Build history of the part. All positions in model axes, mm. Face numbers are marked on the shaded views. A direction names the side the tool comes from. Round coordinates to 2 decimals unless told otherwise and drop trailing zeros. Write each loop counter-clockwise with the first axis right and the second up, starting at its lowest first coordinate (ties: lowest second). Pieces come first, ordered by that corner, then holes. Notation, with made-up numbers: (20.25, -7) - (44.25, -7) arc R33 ccw to (44.25, 30) - close; hole circle Ø2 at (29, -29). An arc over 180 degrees is marked (long way). Answer as a JSON object with one key per item and string values. Group by question number.
Item 1: Flat gauge pins, fed straight in: pin 1 (6 mm diameter, centred on x = -10, y = -7, fed in from +Z); pin 2 (5 mm diameter, centred on x = 11, y = 5, fed in from +Z); pin 3 (12 mm diameter, centred on x = -1, y = -9.5, fed in from +Z). Where does each tip first touch, or does it go through?
Item 2: Two-plate mould, pull along X, no slides. Class the marked faces 1, 2, 3 and 4: +X half, -X half, draft (parallel to the pull), parting line (faces both ways), or undercut.
Item 3: Probe line 1 (X direction, y = 7, z = 1.7); line 2 (Y direction, x = 10, z = 0.95); line 3 (Z direction, x = 0, y = -7.5). List the from-to ranges inside material, lowest first. Write a range as from..to.
Item 4: Slice it at C-C, the plane x = 10. List the corners of the cut face in (y, z), then the cut area to 3 significant figures.
Item 5: Slice it at B-B, the plane x = 0. List the corners of the cut face in (y, z), then the cut area to 3 significant figures.
Item 6: Which spindle directions (+Z, -Z, +X, -X, +Y, -Y) get a long thin tool onto all of the face, cutting with end or side? Do the marked faces 5 and 6. Say none if no direction does.
Item 7: Slice it at D-D, the plane z = 5. List the corners of the cut face in (x, y), then the cut area to 3 significant figures.
Item 8: Slice it at A-A, the plane y = 7. List the corners of the cut face in (x, z), then the cut area to 3 significant figures.
from build123d import *

# Parameters (mm, degrees)
SKETCH_R     = 1.75
PAD_DEPTH    = 15
SKETCH001_R  = 2.25
POCKET_DEPTH = 8.001
FILLET_R     = 4
CHAMFER_SIZE = 1.5


with BuildPart() as part:
    # Sketch → Pad (new body, symmetric)
    with BuildSketch(Plane.XZ):
        with BuildLine():
            Line((20, 4), (20, 0))
            Line((20, 0), (-20, 0))
            Line((-20, 0), (-20, 4))
            Line((-20, 4), (-4, 4))
            ThreePointArc((4, 4), (0, 8), (-4, 4))
            Line((20, 4), (4, 4))
        make_face()
        with Locations((0, 4)):
            Circle(SKETCH_R, mode=Mode.SUBTRACT)
    extrude(amount=PAD_DEPTH, both=True)

    # Sketch001 (on Face2 of Pad) → Pocket (cut, through all)
    with BuildSketch(Plane(origin=(0, 0, 0), x_dir=(1, 0, 0), z_dir=(0, 0, -1))):
        with Locations((10, 7)):
            Circle(SKETCH001_R)
        with Locations((10, -7)):
            Circle(SKETCH001_R)
        with Locations((-10, 7)):
            Circle(SKETCH001_R)
        with Locations((-10, -7)):
            Circle(SKETCH001_R)
    extrude(amount=-POCKET_DEPTH, mode=Mode.SUBTRACT)

    # Fillet
    fillet_edges = [part.edges().sort_by_distance(p)[0] for p in [
        (20, -15, 2),
        (20, 15, 2),
        (-20, 15, 2),
        (-20, -15, 2),
    ]]
    fillet(fillet_edges, radius=FILLET_R)

    # Chamfer
    chamfer_edges = [part.edges().sort_by_distance(p)[0] for p in [
        (-12.25, -7, 4),
        (-12.25, 7, 4),
        (7.75, 7, 4),
        (7.75, -7, 4),
    ]]
    chamfer(chamfer_edges, length=CHAMFER_SIZE)


solid = part.part
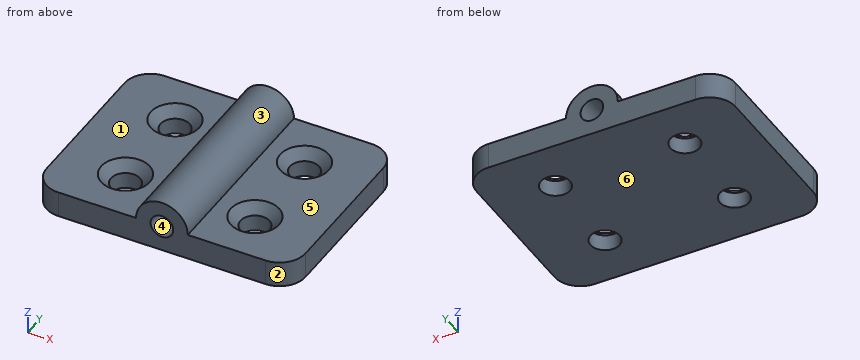
Geometry says:
{
 "1": {"pin 1": "stops at z = 3.25", "pin 2": "stops at z = 4", "pin 3": "stops at z = 8"},
 "2": {"face 1": "draft", "face 2": "+X half", "face 3": "parting line", "face 4": "undercut"},
 "3": {"line 1": "x = -20..-12.25, -7.75..7.75, 12.25..20", "line 2": "y = -15..-9.25, -4.75..4.75, 9.25..15", "line 3": "z = 0..2.25, 5.75..8"},
 "4": {"outline": "(-15, 0) - (-9.25, 0) - (-9.25, 2.5) - (-10.75, 4) - (-15, 4) - close; (-4.75, 0) - (4.75, 0) - (4.75, 2.5) - (3.25, 4) - (-3.25, 4) - (-4.75, 2.5) - close; (9.25, 0) - (15, 0) - (15, 4) - (10.75, 4) - (9.25, 2.5) - close", "area": "79.5 mm^2"},
 "5": {"outline": "(-15, 0) - (15, 0) - (15, 2.25) - (-15, 2.25) - close; (-15, 5.75) - (15, 5.75) - (15, 8) - (-15, 8) - close", "area": "135 mm^2"},
 "6": {"face 5": "+Z, +X, +Y, -Y", "face 6": "-Z, +X, -X, +Y, -Y"},
 "7": {"outline": "(-3.87, -15) - (-1.44, -15) - (-1.44, 15) - (-3.87, 15) - close; (1.44, -15) - (3.87, -15) - (3.87, 15) - (1.44, 15) - close", "area": "146 mm^2"},
 "8": {"outline": "(-20, 0) - (-12.25, 0) - (-12.25, 2.5) - (-13.75, 4) - (-20, 4) - close; (-7.75, 0) - (7.75, 0) - (7.75, 2.5) - (6.25, 4) - (4, 4) arc R4 ccw to (-4, 4) - (-6.25, 4) - (-7.75, 2.5) - close; (12.25, 0) - (20, 0) - (20, 4) - (13.75, 4) - (12.25, 2.5) - close; hole circle Ø3.5 at (0, 4)", "area": "135 mm^2"}
}
